Design review of the part built by this model. Coordinates are the model's own, in mm. A direction names the side the tool comes from. Give positions to 0.01 mm unless a question says otherwise; leave off trailing zeros. Write each loop counter-clockwise with the first axis right and the second up, starting at its lowest first coordinate (ties: lowest second). Pieces come first, ordered by that corner, then holes. Notation, with made-up numbers: (30, 42) -> (46, 42) arc R10 cw to (46, 51) -> close; hole circle Ø2 at (7, 20.25). An arc over 180 degrees is marked (long way). Return JSON: item names as keys, results as strings. Group by question number.
from build123d import *

# Parameters (mm, degrees)
SKETCH_1_W          = 150
SKETCH_1_H          = 150
EXTRUDE_1_DEPTH     = 5
SKETCH_3_W          = 150
SKETCH_3_H          = 150
SKETCH_3_W_2        = 140
SKETCH_3_H_2        = 140
EXTRUDE_2_DEPTH     = 140
SKETCH_5_R          = 1.65
CUT_EXTRUDE_1_DEPTH = 5
SKETCH_8_W          = 150
SKETCH_8_H          = 150
SKETCH_8_R          = 50
EXTRUDE_3_DEPTH     = 5
SKETCH_7_R          = 3
CUT_EXTRUDE_2_DEPTH = 257.953303151


with BuildPart() as part:
    # 草图1 → 凸台-拉伸1 (new body)
    with BuildSketch(Plane(origin=(0, 0, 0), x_dir=(1, 0, 0), z_dir=(0, 1, 0))):
        with Locations((75, 75)):
            Rectangle(SKETCH_1_W, SKETCH_1_H)
    extrude(amount=EXTRUDE_1_DEPTH)

    # 草图3 → 凸台-拉伸2 (add)
    with BuildSketch(Plane.XZ):
        with Locations((75, -75)):
            Rectangle(SKETCH_3_W, SKETCH_3_H)
        with Locations((75, -75)):
            Rectangle(SKETCH_3_W_2, SKETCH_3_H_2, mode=Mode.SUBTRACT)
    extrude(amount=EXTRUDE_2_DEPTH)

    # 草图5 → 切除-拉伸1 (cut)
    with BuildSketch(Plane(origin=(0, 5, 0), x_dir=(1, 0, 0), z_dir=(0, 1, 0))):
        with Locations(Location((75, 115, 0), (0, 0, 270))):
            Circle(SKETCH_5_R)
        with Locations(Location((75, 35, 0), (0, 0, 90))):
            Circle(SKETCH_5_R)
    extrude(amount=-CUT_EXTRUDE_1_DEPTH, mode=Mode.SUBTRACT)

    # 草图8 → 凸台-拉伸3 (add)
    with BuildSketch(Plane.XZ.offset(140)):
        with Locations((75, -75)):
            Rectangle(SKETCH_8_W, SKETCH_8_H)
        with Locations(Location((75, -75, 0), (0, 0, 270))):
            Circle(SKETCH_8_R, mode=Mode.SUBTRACT)
    extrude(amount=EXTRUDE_3_DEPTH)

    # 草图7 → 切除-拉伸2 (cut, through all)
    with BuildSketch(Plane(origin=(150, 0, 0), x_dir=(0, 0, -1), z_dir=(1, 0, 0))):
        with Locations((85.95, -45)):
            Circle(SKETCH_7_R)
    extrude(amount=-CUT_EXTRUDE_2_DEPTH, mode=Mode.SUBTRACT)


solid = part.part
Q1. Take a section at C-C, the plane z = -75. Give the boundary of the cut face in (x, y).
Q2. Tool access review of faces 5 (the face through (74, -69, -145)), 6 (the face through (30.64, -142.46, -98.07)), 7 (the face through (74, -69, 0)): name each direction out of +Z, -Z, +X, -X, +Y, -Y from which nothing blocks a thin tool from reaching the whole face with its end or side.
Q3. For L1, parallel to Z at x = 75, y = 2.8; L2, parallel to Z at x = 51.5, y = -85; L3, parallel to X at y = -134.5, z = -44, list the stretches that pass through material, from the lowest coordinate up. Write a range as from..to.
Q4. Take a section at B-B, the plane y = -35.5. Give the boundary of the cut face in (x, z).
Q5. Insertion check: pin 1 (2 mm diameter, centred on x = 75, z = -115, fed in from -Y). The pin has a flat end and moves straight along its axis. Give the tip position at first contact, or say it passes through.
Q6. Take a section at A-A, the plane x = 141. Give the boundary of the cut face in (y, z), plus the area to 3 significant figures.
Q7. Take a section at D-D, the plane x = 63. Give the boundary of the cut face in (y, z).
Q8. Mouldability with a two-part tool opening along X and no side actions: class faces 1 (the face through (2.53, -42.97, -83.74)), 2 (the face through (0, -69, -76)), 3 (the face through (150, -69, -76)), 4 (the face through (74, -69, -5)) as +X half, -X half, draft (parallel to the pull), parting line (faces both ways), or undercut.
Final values:
{
 "1": {"outline": "(0, -145) -> (25, -145) -> (25, -140) -> (5, -140) -> (5, 0) -> (145, 0) -> (145, -140) -> (125, -140) -> (125, -145) -> (150, -145) -> (150, 5) -> (0, 5) -> close"},
 "2": {"face 5": "none", "face 6": "-Y", "face 7": "+Z, +X, -X, +Y, -Y"},
 "3": {"L1": "z = -150..-116.65, -113.35..-36.65, -33.35..0", "L2": "z = -150..-145, -5..0", "L3": "x = 0..5, 145..150"},
 "4": {"outline": "(0, -150) -> (150, -150) -> (150, 0) -> (0, 0) -> close; hole (5, -145) -> (145, -145) -> (145, -5) -> (5, -5) -> close"},
 "5": {"pin 1": "passes through"},
 "6": {"outline": "(-145, -150) -> (5, -150) -> (5, 0) -> (-145, 0) -> close; hole (-140, -145) -> (0, -145) -> (0, -5) -> (-140, -5) -> close", "area": "2,900 mm²"},
 "7": {"outline": "(-145, -150) -> (5, -150) -> (5, 0) -> (-145, 0) -> (-145, -26.46) -> (-140, -26.46) -> (-140, -5) -> (0, -5) -> (0, -145) -> (-140, -145) -> (-140, -123.54) -> (-145, -123.54) -> close"},
 "8": {"face 1": "draft", "face 2": "-X half", "face 3": "+X half", "face 4": "undercut"}
}
